```python
from build123d import *

# Parameters (mm, degrees)
SKETCH1_R           = 4
SKETCH1_R_2         = 2
SKETCH1_R_3         = 3
SKETCH1_R_4         = 1.5
BOSS_EXTRUDE1_DEPTH = 1.5


with BuildPart() as part:
    # Sketch1 → Boss-Extrude1 (new, symmetric)
    # profile 1 of 3: a face of its own
    with BuildSketch(Plane(origin=(0, 0, 0), x_dir=(1, 0, 0), z_dir=(0, 1, 0))):
        with BuildLine():
            Line((-11.5, 4), (-17.5, 4))
            ThreePointArc((-17.5, 4), (-14.671572875, 2.828427125), (-13.5, 0))
            ThreePointArc((-13.5, 0), (-14.671572875, -2.828427125), (-17.5, -4))
            Line((-17.5, -4), (-11.5, -4))
            ThreePointArc((-11.5, -4), (-8.632069519, -2.34904785), (-5.341350168, -2))
            Line((-5.341350168, -2), (6.516979908, -2))
            ThreePointArc((6.516979908, -2), (9.090013088, -2.093768583), (11.5, -3))
            Line((11.5, -3), (17.5, -3))
            ThreePointArc((17.5, -3), (14.5, 0), (17.5, 3))
            Line((17.5, 3), (11.5, 3))
            ThreePointArc((11.5, 3), (9.090013088, 2.093768583), (6.516979908, 2))
            Line((6.516979908, 2), (-5.341350168, 2))
            ThreePointArc((-5.341350168, 2), (-8.632069519, 2.34904785), (-11.5, 4))
        make_face()
    # profile 2 of 3: a face of its own
    with BuildSketch(Plane(origin=(0, 0, 0), x_dir=(1, 0, 0), z_dir=(0, 1, 0))):
        with Locations((-17.5, 0)):
            Circle(SKETCH1_R)
        with Locations(Location((-17.5, 0, 0), (0, 0, 270))):
            Circle(SKETCH1_R_2, mode=Mode.SUBTRACT)
    # profile 3 of 3: a face of its own
    with BuildSketch(Plane(origin=(0, 0, 0), x_dir=(1, 0, 0), z_dir=(0, 1, 0))):
        with Locations((17.5, 0)):
            Circle(SKETCH1_R_3)
        with Locations(Location((17.5, 0, 0), (0, 0, 270))):
            Circle(SKETCH1_R_4, mode=Mode.SUBTRACT)
    extrude(amount=BOSS_EXTRUDE1_DEPTH, both=True)


solid = part.part
```
Model file for the job. Use its own axes, mm. A direction names the side the tool comes from. Coordinates: 2 decimals unless noted, no trailing zeros. Loops run counter-clockwise (first coordinate to the right, second up) from the corner with the lowest first, then second, coordinate; pieces in that order, holes last. Notation, with made-up numbers: (62.5, 69.5) - (111.5, 69.5) arc R13 ccw to (111.5, 83.5) - close; hole circle Ø8 at (81.5, -13). An arc over 180 degrees is marked (long way). Answer as a JSON object with one key per item and string values. Group by question number.
(1) Tool access for faces 1 (the face through (-1, 1.5, 0)), 2 (the face through (15, 0, -3)): list every direction of +Z, -Z, +X, -X, +Y, -Y with a clear straight run to the whole face (end or side of a thin tool).
(2) Cut at B-B (z = 0). Give the cut face in (x, y), then the cut area to 3 significant figures.
(3) Cut at C-C (x = -3). Give the cut face in (y, z), then the cut area to 3 significant figures.
(4) Flat gauge pins, fed straight in: pin 1 (0.8 mm diameter, centred on x = 15, y = -1, fed in from +Z); pin 2 (1 mm diameter, centred on y = 0.5, z = 2.5, fed in from -X); pin 3 (1.5 mm diameter, centred on x = 13, y = 0.5, fed in from -Z). Where does each tip first touch, or does it go through?
(5) Cut at A-A (y = 0.9). Give the cut face in (x, z).
(6) Probe line 1 along X through (y, z) = (-0.4, 0); line 2 along Z through (x, y) = (8.5, -1.35); line 3 along Z through (x, y) = (13, 0.85). List the from-to ranges inside material, lowest first.
(7) Two-plate mould, pull along X, no slides. Class faces 3 (the face through (9.13, 0.02, -2.1)), 4 (the face through (20.5, 0, 0.1)), 5 (the face through (-1, -1.5, 0)): released by +X, released by -X, zero draft, split by the parting line, or undercut.
Geometry says:
{
 "1": {"face 1": "+Z, -Z, +X, -X, +Y", "face 2": "-Z, +X, +Y, -Y"},
 "2": {"outline": "(-21.5, -1.5) - (-19.5, -1.5) - (-19.5, 1.5) - (-21.5, 1.5) - close; (-15.5, -1.5) - (16, -1.5) - (16, 1.5) - (-15.5, 1.5) - close; (19, -1.5) - (20.5, -1.5) - (20.5, 1.5) - (19, 1.5) - close", "area": "105 mm^2"},
 "3": {"outline": "(-1.5, -2) - (1.5, -2) - (1.5, 2) - (-1.5, 2) - close", "area": "12.0 mm^2"},
 "4": {"pin 1": "stops at z = 3", "pin 2": "stops at x = -20.96", "pin 3": "stops at z = -3"},
 "5": {"outline": "(-17.5, -4) - (-11.5, -4) arc R8 cw to (-5.34, -2) - (6.52, -2) arc R8 cw to (11.5, -3) - (17.5, -3) arc R3 ccw to (17.5, 3) - (11.5, 3) arc R8 cw to (6.52, 2) - (-5.34, 2) arc R8 cw to (-11.5, 4) - (-17.5, 4) arc R4 ccw to start; hole circle Ø4 at (-17.5, 0); hole circle Ø3 at (17.5, 0)"},
 "6": {"line 1": "x = -21.5 to -19.5, -15.5 to 16, 19 to 20.5", "line 2": "z = -2 to 2", "line 3": "z = -3 to 3"},
 "7": {"face 3": "undercut", "face 4": "released by +X", "face 5": "zero draft"}
}
